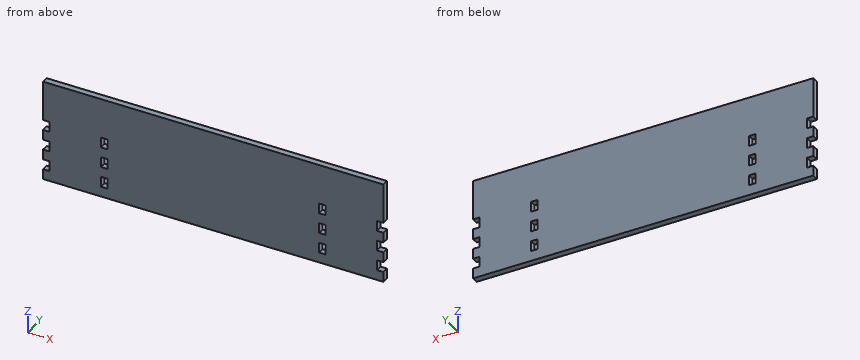
```python
from build123d import *

# Parameters (mm, degrees)
SKETCH1_W           = 3.175
SKETCH1_H           = 5
BOSS_EXTRUDE1_DEPTH = 3.175


with BuildPart() as part:
    # Sketch1 → Boss-Extrude1 (new body)
    with BuildSketch(Plane(origin=(0, 0, 0), x_dir=(1, 0, 0), z_dir=(0, 1, 0))):
        Polygon((-167.9575, -5), (-164.7825, -5), (-164.7825, -10), (-167.9575, -10), (-167.9575, -15), (-164.7825, -15), (-164.7825, -20), (-167.9575, -20), (-167.9575, -25), (-164.7825, -25), (-164.7825, -30), (-167.9575, -30), (-167.9575, -49.53), (-164.7825, -49.53), (-66.4845, -49.53), (0, -49.53), (0, -30), (-3.175, -30), (-3.175, -25), (0, -25), (0, -20), (-3.175, -20), (-3.175, -15), (0, -15), (0, -10), (-3.175, -10), (-3.175, -5), (0, -5), (0, 0), (-66.4845, 0), (-164.7825, 0), (-167.9575, 0), align=None)
        with Locations((-137.795, -7.5)):
            Rectangle(SKETCH1_W, SKETCH1_H, mode=Mode.SUBTRACT)
        with Locations((-137.795, -17.5)):
            Rectangle(SKETCH1_W, SKETCH1_H, mode=Mode.SUBTRACT)
        with Locations((-137.795, -27.5)):
            Rectangle(SKETCH1_W, SKETCH1_H, mode=Mode.SUBTRACT)
        with Locations((-30.1625, -27.5)):
            Rectangle(SKETCH1_W, SKETCH1_H, mode=Mode.SUBTRACT)
        with Locations((-30.1625, -17.5)):
            Rectangle(SKETCH1_W, SKETCH1_H, mode=Mode.SUBTRACT)
        with Locations((-30.1625, -7.5)):
            Rectangle(SKETCH1_W, SKETCH1_H, mode=Mode.SUBTRACT)
    extrude(amount=BOSS_EXTRUDE1_DEPTH)


solid = part.part
```
The listing builds one solid part. Answer for the finished solid, in the listing's coordinates (mm). Give positions to 0.01 mm unless a question says otherwise; leave off trailing zeros. Answer as CSV lines item,"result". Start each with the question number.
Q1. Find the intervals of material crossed by L1, parallel to Z at x = -29.5, y = 2.3, in increasing order.
Q2. A cutting plane is placed at A-A (z = 8). Count the separate pieces of the cut face and the enclosed holes in it, then the cut area to 3 significant figures.
Q3. Given pin 1 (1 mm diameter, centred on y = 1, z = 27, fed in from +X) (3 decimals); pin 2 (1.6 mm diameter, centred on x = -2, y = 1, fed in from -Z); pin 3 (1.6 mm diameter, centred on y = 1.5, z = 7, fed in from -X), each flat-ended and moving along its own axis, determine where each tip first touches the part or whether it passes through.
Results found:
1,L1,"0 to 5, 10 to 15, 20 to 25, 30 to 49.53"
2,separate pieces,"3"
2,enclosed holes,"0"
2,area,"493 mm2"
3,pin 1,"x = -3.175"
3,pin 2,"z = 0"
3,pin 3,"x = -164.78"
